Could you check a few things on this model? Use its own coordinates, in mm. A direction names the side the tool comes from. Round coordinates to 2 decimals unless told otherwise and drop trailing zeros. Write each loop counter-clockwise with the first axis right and the second up, starting at its lowest first coordinate (ties: lowest second). Pieces come first, ordered by that corner, then holes. Notation, with made-up numbers: (24.5, 47) -> (73.5, 47) arc R20 ccw to (73.5, 66) -> close; hole circle Ø6 at (57.5, 15.5). An arc over 180 degrees is marked (long way). Answer in a Markdown table with one row per item. Add a question column.
```python
from build123d import *

# Parameters (mm, degrees)
SKETCH_1_R      = 1.75
SKETCH_1_W      = 3
SKETCH_1_H      = 7.5
EXTRUDE_1_DEPTH = 5


with BuildPart() as part:
    # Эскиз1 → Бобышка-Вытянуть1 (new body)
    with BuildSketch(Plane(origin=(0, 0, 0), x_dir=(0, 0, -1), z_dir=(1, 0, 0))):
        Polygon((-36.75, 45), (-36.75, 42.5), (-39.25, 42.5), (-39.25, 40), (-30.75, 40), (-30.75, 42.5), (-33.25, 42.5), (-33.25, 45), (33.25, 45), (33.25, 42.5), (30.75, 42.5), (30.75, 40), (39.25, 40), (39.25, 42.5), (36.75, 42.5), (36.75, 45), (50, 45), (50, -45), (36.75, -45), (36.75, -42.5), (39.25, -42.5), (39.25, -40), (30.75, -40), (30.75, -42.5), (33.25, -42.5), (33.25, -45), (-33.25, -45), (-33.25, -42.5), (-30.75, -42.5), (-30.75, -40), (-39.25, -40), (-39.25, -42.5), (-36.75, -42.5), (-36.75, -45), (-50, -45), (-50, 45), align=None)
        with Locations((-47, 30)):
            Circle(SKETCH_1_R, mode=Mode.SUBTRACT)
        with Locations((47, 30)):
            Circle(SKETCH_1_R, mode=Mode.SUBTRACT)
        with Locations((47, -30)):
            Circle(SKETCH_1_R, mode=Mode.SUBTRACT)
        with Locations((-47, -30)):
            Circle(SKETCH_1_R, mode=Mode.SUBTRACT)
        with Locations((-30, -22.5)):
            Circle(SKETCH_1_R, mode=Mode.SUBTRACT)
        with Locations((30, -22.5)):
            Circle(SKETCH_1_R, mode=Mode.SUBTRACT)
        with Locations((8.5, -10)):
            Rectangle(SKETCH_1_W, SKETCH_1_H, mode=Mode.SUBTRACT)
        with Locations((-8.5, -10)):
            Rectangle(SKETCH_1_W, SKETCH_1_H, mode=Mode.SUBTRACT)
    extrude(amount=EXTRUDE_1_DEPTH)


solid = part.part
```
(1) Suppose I cut it at A-A, the plane z = -47. Please give me the cut outline in (x, y), then the cut area to 3 significant figures.
(2) Suppose I cut it at C-C, the plane x = 4.2. State how many separate pieces and enclosed holes the cut face has, then the cut area to 3 significant figures.
(3) For P1, Ø4.5, axis at y = -30, z = -47, coming from the -X side, with a flat end and sliding along its axis, tell me the tip position at first contact or that it passes through.
(4) I need wall thicknesses on L1, parallel to Z at x = 2.15, y = -7; L2, parallel to Y at x = 0.95, z = -32; L3, parallel to Y at x = 3.6, z = -47. Which ranges of each line are inside material? Lowest first, please.
(5) If we mould it in two halves opening along Y, with no side actions, what happens to faces 1 (the face through (2, -45, 0)), 2 (the face through (2, -44, -33.25)), 3 (the face through (2, 41, 39.25))? For each: pulls with the +Y half, pulls with the -Y half, needs draft (parallel to the pull), parting line crosses it, or undercut.
(6) Suppose I cut it at B-B, the plane y = -30. Please give me the cut outline in (x, z), then the cut area to 3 significant figures.
(7) On a 3-axis mill with a long thin cutter (end or side, diameter ignored), from which of +Z, -Z, +X, -X, +Y, -Y can I reach the whole of each face in a straight line? I mean faces 4 (the face through (2, -44, 36.75)), 5 (the face through (2, 44, -33.25)), 6 (the face through (2, 42.5, 32)). Say none if no direction works.
Response:
| question | item | result |
|---|---|---|
| 1 | outline | (0, -45) -> (5, -45) -> (5, -31.75) -> (0, -31.75) -> close; (0, -28.25) -> (5, -28.25) -> (5, 28.25) -> (0, 28.25) -> close; (0, 31.75) -> (5, 31.75) -> (5, 45) -> (0, 45) -> close |
| 1 | area | 415 mm² |
| 2 | separate pieces | 1 |
| 2 | enclosed holes | 8 |
| 2 | area | 8,780 mm² |
| 3 | P1 | x = 0 |
| 4 | L1 | -50 to -10, -7 to 7, 10 to 50 |
| 4 | L2 | -45 to -42.5, -40 to 40, 42.5 to 45 |
| 4 | L3 | -45 to -31.75, -28.25 to 28.25, 31.75 to 45 |
| 5 | face 1 | pulls with the -Y half |
| 5 | face 2 | needs draft |
| 5 | face 3 | undercut |
| 6 | outline | (0, -50) -> (5, -50) -> (5, -48.75) -> (0, -48.75) -> close; (0, -45.25) -> (5, -45.25) -> (5, 45.25) -> (0, 45.25) -> close; (0, 48.75) -> (5, 48.75) -> (5, 50) -> (0, 50) -> close |
| 6 | area | 465 mm² |
| 7 | face 4 | +X, -X, -Y |
| 7 | face 5 | +X, -X, +Y |
| 7 | face 6 | +X, -X |
